```python
from build123d import *

# Parameters (mm, degrees)
SKETCH1_W           = 190.2
SKETCH1_H           = 30
BOSS_EXTRUDE1_DEPTH = 3.2
SKETCH2_R           = 1.75
CUT_EXTRUDE1_DEPTH  = 97.328863795
SKETCH3_R           = 3.25
CUT_EXTRUDE2_DEPTH  = 97.328863795
FILLET1_R           = 5


with BuildPart() as part:
    # Sketch1 → Boss-Extrude1 (new body)
    with BuildSketch(Plane(origin=(0, 0, 0), x_dir=(1, 0, 0), z_dir=(0, 1, 0))):
        Rectangle(SKETCH1_W, SKETCH1_H)
    extrude(amount=BOSS_EXTRUDE1_DEPTH)

    # Sketch2 → Cut-Extrude1 (cut, through all)
    with BuildSketch(Plane(origin=(0, 3.2, 0), x_dir=(1, 0, 0), z_dir=(0, 1, 0))):
        with Locations(Location((-90, 10, 0), (0, 0, 270))):
            Circle(SKETCH2_R)
        with Locations(Location((-90, -10, 0), (0, 0, 270))):
            Circle(SKETCH2_R)
        with Locations(Location((90, 10, 0), (0, 0, 270))):
            Circle(SKETCH2_R)
        with Locations(Location((90, -10, 0), (0, 0, 270))):
            Circle(SKETCH2_R)
    extrude(amount=-CUT_EXTRUDE1_DEPTH, mode=Mode.SUBTRACT)

    # Sketch3 → Cut-Extrude2 (cut, through all)
    with BuildSketch(Plane(origin=(0, 3.2, 0), x_dir=(1, 0, 0), z_dir=(0, 1, 0))):
        with Locations(Location((65.7, -10.1, 0), (0, 0, 270))):
            Circle(SKETCH3_R)
        with Locations(Location((27.6, -10.1, 0), (0, 0, 270))):
            Circle(SKETCH3_R)
        with Locations(Location((-27.6, -10.1, 0), (0, 0, 270))):
            Circle(SKETCH3_R)
        with Locations(Location((-65.7, -10.1, 0), (0, 0, 270))):
            Circle(SKETCH3_R)
    extrude(amount=-CUT_EXTRUDE2_DEPTH, mode=Mode.SUBTRACT)

    # Fillet1
    fillet1_edges = [part.edges().sort_by_distance(p)[0] for p in [
        (95.1, 1.6, 15),
        (-95.1, 1.6, 15),
        (-95.1, 1.6, -15),
        (95.1, 1.6, -15),
    ]]
    fillet(fillet1_edges, radius=FILLET1_R)


solid = part.part
```
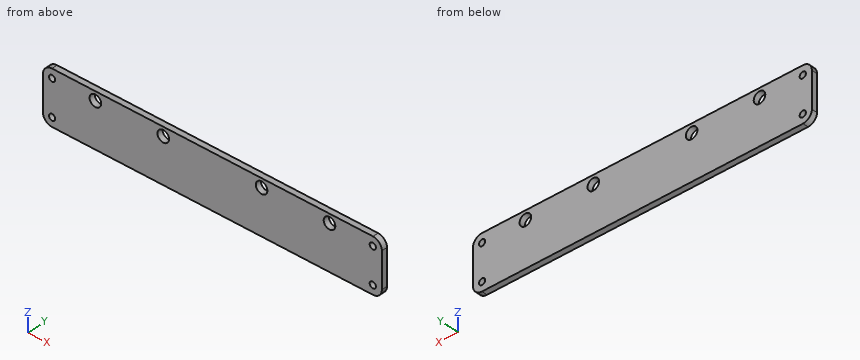
Read the model definition and answer for the solid it produces. Units are mm, in the model's axes. Round coordinates to 2 decimals unless told otherwise and drop trailing zeros. Write each loop counter-clockwise with the first axis right and the second up, starting at its lowest first coordinate (ties: lowest second). Pieces come first, ordered by that corner, then holes. Notation, with made-up numbers: (-39.5, -29) -> (0.5, -29) arc R20 ccw to (0.5, 3) -> close; hole circle Ø6 at (62, -12). An arc over 180 degrees is marked (long way). Answer in a Markdown table with one row per item. Add a question column.
1) Consider line 1 (Z direction, x = -90, y = 1.45); line 2 (X direction, y = 1.6, z = -9.75); line 3 (X direction, y = 0.2, z = -8.75). Determine where each line is inside the solid, lowest interval first.
2) Find section A-A, the plane x = -65.7. Determine the outline of the cut face in (y, z), and give its area (3 significant figures).
3) Find section B-B, the plane y = 2.55. State how many separate pieces and enclosed holes the cut face has, and give its area (3 significant figures).
Findings below:
| question | item | result |
|---|---|---|
| 1 | line 1 | -15 to -11.75, -8.25 to 8.25, 11.75 to 15 |
| 1 | line 2 | -95.1 to -91.73, -88.27 to 88.27, 91.73 to 95.1 |
| 1 | line 3 | -95.1 to -91.22, -88.78 to 88.78, 91.22 to 95.1 |
| 2 | outline | (0, -15) -> (3.2, -15) -> (3.2, 6.85) -> (0, 6.85) -> close; (0, 13.35) -> (3.2, 13.35) -> (3.2, 15) -> (0, 15) -> close |
| 2 | area | 75.2 mm² |
| 3 | separate pieces | 1 |
| 3 | enclosed holes | 8 |
| 3 | area | 5,510 mm² |
